Read the model definition and answer for the solid it produces. Units are mm, in the model's axes. A direction names the side the tool comes from. Give positions to 0.01 mm unless a question says otherwise; leave off trailing zeros. Loops run counter-clockwise (first coordinate to the right, second up) from the corner with the lowest first, then second, coordinate; pieces in that order, holes last.
(1) Each of these flat-tipped pins is pushed along its axis until it touches: P1, Ø2, axis at x = 1.5, y = 12, coming from the +Z side; P2, Ø4.5, axis at x = 0, z = 0, coming from the +Y side; P3, Ø3, axis at x = 0, y = 0, coming from the -Z side; P4, Ø3.5, axis at y = 10, z = 10, coming from the +X side. Where does it stop, or does it pass through?
(2) Find section C-C, the plane x = 0. State how many separate pieces and enclosed holes the cut face has, then the cut area to 3 significant figures.
(3) Find section A-A, the plane z = -10. Write down the section's boundary in (x, y), then the cut area to 3 significant figures.
(4) Which of the six approach directions +Z, -Z, +X, -X, +Y, -Y give full straight-line access (tool end or side, diameter ignored) to faces 4 (the face through (4.25, 1.34, 16.1)), 5 (the face through (-1.073, 16.925, 4.832)), 6 (the face through (-0.077, -8.581, -8.452)), 7 (the face through (-1.073, -4.832, 16.925))?
(5) Find section B-B, the plane y = 10. Write down the section's boundary in (x, z), then the cut area to 3 significant figures.
(6) Straight lines are drawn through the part: probe 1 along Y at (x, z) = (-0.5, 10); probe 2 along Y at (x, z) = (-1.75, -13); probe 3 along Z at (x, y) = (0, -12.5). For each, find the intervals that lie inside material, in ascending order.
(7) Determine the mould class of faces 1 (the face through (4.72, -1.49, -16.92)), 2 (the face through (0, 6, 12.1)), 3 (the face through (0, -12.1, -6)) for opening direction Z: pulls with the +Z half, pulls with the -Z half, needs draft (parallel to the pull), parting line crosses it, or undercut.
```python
from build123d import *
from build123d.topology import SkipClean

# Parameters (mm, degrees)
CIRPATTERN1_COUNT     = 4
CIRPATTERN2_COUNT     = 4
SKETCH4_R             = 3.624
SKETCH4_R_2           = 2.1
BOSS_EXTRUDE1_DEPTH   = 5.5
BOSS_EXTRUDE1_2_DEPTH = 5.5
BOSS_EXTRUDE2_DEPTH   = 1.833333333


with BuildPart() as part:
    # Sketch1 → Revolve1 (revolve)
    with BuildSketch(Plane(origin=(0, 0, 0), x_dir=(0, 0, -1), z_dir=(1, 0, 0)), mode=Mode.PRIVATE) as revolve1_sk:
        with BuildLine():
            Line((16.603, 4.95), (17.238, 4.95))
            ThreePointArc((17.238, 4.95), (17.776815367, 4.726815367), (18, 4.188))
            Line((18, 4.188), (18, 2.381))
            Line((18, 2.381), (17.619, 2))
            Line((17.619, 2), (7.714285714, 2))
            Line((7.714285714, 2), (7.714285714, 1.238))
            Line((7.714285714, 1.238), (0, 1.238))
            Line((0, 1.238), (0, 4.4))
            Line((0, 4.4), (5.4, 4.4))
            Line((5.4, 4.4), (7.305255888, 5.5))
            Line((7.305255888, 5.5), (15.587, 5.5))
            Line((15.587, 5.5), (15.587, 4.455))
            Line((15.587, 4.455), (16.603, 4.455))
            Line((16.603, 4.455), (16.603, 4.95))
        make_face()
    revolve(revolve1_sk.sketch.rotate(Axis((0, 0, 0), (0, 0, -1)), 90), axis=Axis((0, 0, 0), (0, 0, -1)))


with BuildPart() as cirpattern1_1:
    # CirPattern1: pattern copy
    add(part.part.rotate(Axis((0, 0, 0), (1, 0, 0)), 1 * 360 / CIRPATTERN1_COUNT))


with BuildPart() as cirpattern1_2:
    # CirPattern1: pattern copy
    add(part.part.rotate(Axis((0, 0, 0), (1, 0, 0)), 2 * 360 / CIRPATTERN1_COUNT))


with BuildPart() as cirpattern1_3:
    # CirPattern1: pattern copy
    add(part.part.rotate(Axis((0, 0, 0), (1, 0, 0)), 3 * 360 / CIRPATTERN1_COUNT))


with BuildPart() as part_1:
    add(part.part)

    # Combine1: union CirPattern1_1, CirPattern1_2, CirPattern1_3
    add(cirpattern1_1.part)
    add(cirpattern1_2.part)
    add(cirpattern1_3.part)

    # Sketch3 → Cut-Revolve1 (revolve, cut)
    with BuildSketch(Plane(origin=(0, 0, 0), x_dir=(0, 0, -1), z_dir=(1, 0, 0)), mode=Mode.PRIVATE) as cut_revolve1_sk:
        Polygon((18, 2.381), (17.619, 2), (7.714285714, 2), (7.714285714, 1.238), (0, 1.238), (0, 0), (18, 0), align=None)
    cut_revolve1 = revolve(cut_revolve1_sk.sketch.rotate(Axis((0, 0, 0), (0, 0, -1)), 90), axis=Axis((0, 0, 0), (0, 0, -1)), mode=Mode.SUBTRACT)

    # CirPattern2: Cut-Revolve1 ×4 about axis
    cirpattern2_axis = Axis((-6.05, 0, 0), (1, 0, 0))
    for i in range(1, CIRPATTERN2_COUNT):
        add(cut_revolve1.rotate(cirpattern2_axis, i * 360 / CIRPATTERN2_COUNT), mode=Mode.SUBTRACT)



with BuildPart() as body_2:
    # Sketch4 → Boss-Extrude1 (new, symmetric)
    with BuildSketch(Plane(origin=(0, 0, 0), x_dir=(0, 0, -1), z_dir=(1, 0, 0))):
        with Locations((-10, 10)):
            Circle(SKETCH4_R)
        with Locations((-10, 10)):
            Circle(SKETCH4_R_2, mode=Mode.SUBTRACT)
    extrude(amount=BOSS_EXTRUDE1_DEPTH, both=True)


with BuildPart() as body_3:
    # Sketch4 → Boss-Extrude1 2 (new, symmetric)
    with BuildSketch(Plane(origin=(0, 0, 0), x_dir=(0, 0, -1), z_dir=(1, 0, 0))):
        with Locations((10, -10)):
            Circle(SKETCH4_R)
        with Locations((10, -10)):
            Circle(SKETCH4_R_2, mode=Mode.SUBTRACT)
    extrude(amount=BOSS_EXTRUDE1_2_DEPTH, both=True)


with BuildPart() as part_2:
    with SkipClean():  # the faces are left unmerged after this step: merging them gives an invalid solid
        add(part_1.part)

        add(body_2.part)  # Boss-Extrude2 merges body 2

        add(body_3.part)  # Boss-Extrude2 merges body 3
        # Sketch5 → Boss-Extrude2 (add, symmetric)
        with BuildSketch(Plane(origin=(0, 0, 0), x_dir=(0, 0, -1), z_dir=(1, 0, 0))):
            with BuildLine():
                Line((10, -12.1), (2, -12.1))
                Line((2, -12.1), (2, -7.9))
                Line((2, -7.9), (7.9, -7.9))
                Line((7.9, -7.9), (7.9, -2))
                Line((7.9, -2), (12.1, -2))
                Line((12.1, -2), (12.1, -10))
                ThreePointArc((12.1, -10), (8.51507576, -8.51507576), (10, -12.1))
            make_face()
            with BuildLine():
                Line((-10, 12.1), (-2, 12.1))
                Line((-2, 12.1), (-2, 7.9))
                Line((-2, 7.9), (-7.9, 7.9))
                Line((-7.9, 7.9), (-7.9, 2))
                Line((-7.9, 2), (-12.1, 2))
                Line((-12.1, 2), (-12.1, 10))
                ThreePointArc((-12.1, 10), (-8.51507576, 8.51507576), (-10, 12.1))
            make_face()
        extrude(amount=BOSS_EXTRUDE2_DEPTH, both=True)


solid = part_2.part
```
Entries:
1. P1: stops at z = 13.48
1. P2: stops at y = 17.87
1. P3: stops at z = -7.71
1. P4: passes through
2. separate pieces: 4
2. enclosed holes: 4
2. area: 481 mm2
3. outline: (-5.5, -13.62) - (5.5, -13.62) - (5.5, -12.1) - (-5.5, -12.1) - close; (-5.5, -7.9) - (5.5, -7.9) - (5.5, -6.38) - (1.83, -6.38) - (1.83, -5.19) arc R5.5 ccw (long way) to (-1.83, -5.19) - (-1.83, -6.38) - (-5.5, -6.38) - close; hole circle Ø4 at (0, 0)
3. area: 120 mm2
4. face 4: none
4. face 5: +Y
4. face 6: +X, -X
4. face 7: +Z
5. outline: (-5.5, 6.38) - (-1.83, 6.38) - (-1.83, 5.19) arc R5.5 ccw (long way) to (1.83, 5.19) - (1.83, 6.38) - (5.5, 6.38) - (5.5, 7.9) - (-5.5, 7.9) - close; (-5.5, 12.1) - (5.5, 12.1) - (5.5, 13.62) - (-5.5, 13.62) - close; hole circle Ø4 at (0, 0)
5. area: 120 mm2
6. probe 1: y = -5.48 to -1.94, 1.94 to 7.9, 12.1 to 13.62
6. probe 2: y = -12.03 to -7.97, -5.21 to -0.97, 0.97 to 5.21
6. probe 3: z = -12.62 to -7.38, -5.5 to -2, 2 to 5.5
7. face 1: needs draft
7. face 2: pulls with the +Z half
7. face 3: undercut
